from build123d import *

# Parameters (mm, degrees)
F3_DEPTH = 50.8
F4_DEPTH = 22.225


with BuildPart() as f2:
    # F1 (on Front) → F2 (revolve)
    with BuildSketch(Plane.XZ):
        Polygon((0, 69.85), (0, 0), (19.177, 0), (16.1234308034, 3.1421328895), (4.7625, 4.9503548071), (4.7625, 69.85), align=None)
    revolve(axis=Axis((0, 0, 0), (0, 0, 1)))

    # F3 (add): a face of the model
    f3_faces = [f2.faces().sort_by_distance(p)[0] for p in [
        (0, 0, 69.85),
    ]]
    extrude(f3_faces, amount=F3_DEPTH)

    # F4 (cut): a face of the model
    f4_faces = [f2.faces().sort_by_distance(p)[0] for p in [
        (0, 0, 120.65),
    ]]
    extrude(f4_faces, amount=-F4_DEPTH, mode=Mode.SUBTRACT)


solid = f2.part
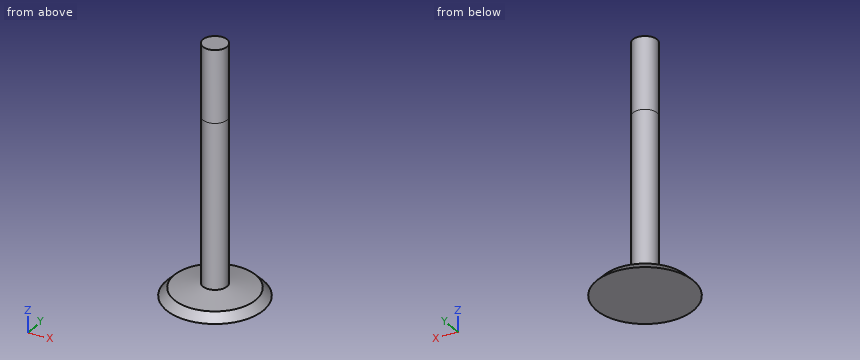
The model under review builds one solid part; all positions refer to its coordinate system, in mm. Round coordinates to 2 decimals unless told otherwise and drop trailing zeros. Write each loop counter-clockwise with the first axis right and the second up, starting at its lowest first coordinate (ties: lowest second). Pieces come first, ordered by that corner, then holes. Notation, with made-up numbers: M 26,51 L 31,51 A21 ccw 31,89 Z; hole C 53,13 d7. An arc over 180 degrees is marked long. Use a Markdown table: item, result. Add a question column.
Q1. We need section C-C, the plane z = 77.5. State the section outline as (x, y) points (1 decimal).
Q2. To check wall thickness, follow line 1 (X direction, y = -2.5, z = 10.5); line 2 (Z direction, x = 0, y = 17); line 3 (Z direction, x = -9.5, y = -14). State the ranges of each line that lie inside material, in increasing order.
Q3. We need section A-A, the plane x = 0. State the section outline as (y, z) points (1 decimal), plus the area to 3 significant figures.
Q4. Insertion check: pin 1 (10 mm diameter, centred on x = -14, y = 3, fed in from +Z); pin 2 (5 mm diameter, centred on x = 6.5, z = 32.5, fed in from -Y); pin 3 (6 mm diameter, centred on x = 10, z = 55.5, fed in from +Y); pin 4 (6 mm diameter, centred on x = -14, y = 6.5, fed in from -Z). Each pin has a flat end and moves straight along its axis. Give the tip position at first contact, or say it passes through.
Findings below:
| question | item | result |
|---|---|---|
| 1 | outline | C 0,0 d9.5 |
| 2 | line 1 | x = -4.05 to 4.05 |
| 2 | line 2 | z = 0 to 2.24 |
| 2 | line 3 | z = 0 to 2.32 |
| 3 | outline | M -19.2,0 L 19.2,0 L 16.1,3.1 L 4.8,5 L 4.8,98.4 L -4.8,98.4 L -4.8,5 L -16.1,3.1 Z |
| 3 | area | 1,040 mm² |
| 4 | pin 1 | stops at z = 4.23 |
| 4 | pin 2 | stops at y = -2.58 |
| 4 | pin 3 | passes through |
| 4 | pin 4 | stops at z = 0 |
